Input: part model. Units: mm. Frame: model coordinates. Face numbers are marked on the shaded views. A direction names the side the tool comes from. Coordinates: 2 decimals unless noted, no trailing zeros. Write each loop counter-clockwise with the first axis right and the second up, starting at its lowest first coordinate (ties: lowest second). Pieces come first, ordered by that corner, then holes. Notation, with made-up numbers: M -24.5,-33.75 L -0.5,-33.75 A21 cw -0.5,4.25 Z; hole C 36,-36 d7. An arc over 180 degrees is marked long. Use one line per item in the form item = value.
from build123d import *

# Parameters (mm, degrees)
SKETCH1_R           = 3.1
SKETCH1_W           = 5.9
SKETCH1_H           = 5.9
BOSS_EXTRUDE1_DEPTH = 3.8
SKETCH2_W           = 5.9
SKETCH2_H           = 5.9
SKETCH2_R           = 1.7
BOSS_EXTRUDE2_DEPTH = 2
SKETCH3_R           = 3.1
BOSS_EXTRUDE3_DEPTH = 2
CHAMFER1_SIZE       = 0.5


with BuildPart() as part:
    # Sketch1 → Boss-Extrude1 (new body)
    with BuildSketch(Plane(origin=(0, 0, 0), x_dir=(1, 0, 0), z_dir=(0, 1, 0))):
        with BuildLine():
            Line((-5, 6.1), (5, 6.1))
            ThreePointArc((5, 6.1), (11.1, 0), (5, -6.1))
            Line((5, -6.1), (-5, -6.1))
            ThreePointArc((-5, -6.1), (-11.1, 0), (-5, 6.1))
        make_face()
        with Locations(Location((5, 0, 0), (0, 0, 90))):
            Circle(SKETCH1_R, mode=Mode.SUBTRACT)
        with Locations((-5, 0)):
            Rectangle(SKETCH1_W, SKETCH1_H, mode=Mode.SUBTRACT)
    extrude(amount=BOSS_EXTRUDE1_DEPTH)

    # Sketch2 → Boss-Extrude2 (add)
    with BuildSketch(Plane(origin=(0, 3.8, 0), x_dir=(1, 0, 0), z_dir=(0, 1, 0))):
        with Locations((-5, 0)):
            Rectangle(SKETCH2_W, SKETCH2_H)
        with Locations(Location((-5, 0, 0), (0, 0, 270))):
            Circle(SKETCH2_R, mode=Mode.SUBTRACT)
    extrude(amount=-BOSS_EXTRUDE2_DEPTH)

    # Sketch3 → Boss-Extrude3 (add)
    with BuildSketch(Plane.XZ):
        with Locations(Location((5, 0, 0), (0, 0, 270))):
            Circle(SKETCH3_R)
    extrude(amount=-BOSS_EXTRUDE3_DEPTH)

    # Chamfer1
    chamfer1_edges = [part.edges().sort_by_distance(p)[0] for p in [
        (5, 3.8, 3.1),
    ]]
    chamfer(chamfer1_edges, length=CHAMFER1_SIZE)


solid = part.part
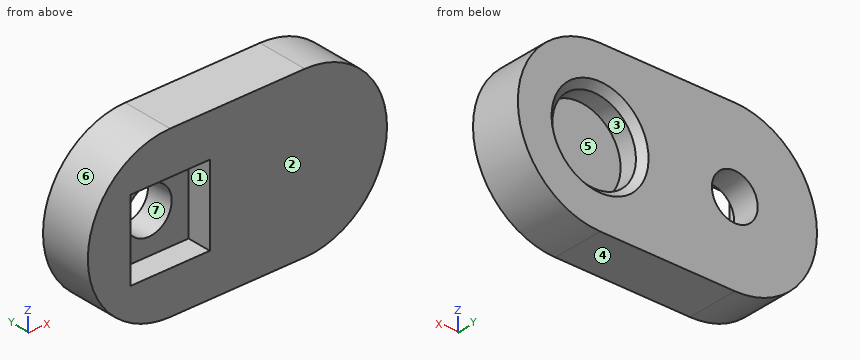
(1) Section query A-A on z = 0. Return the cut outline in (x, y), plus the area to 3 significant figures.
Computed:
outline = M -11.1,0 L -7.95,0 L -7.95,1.8 L -6.7,1.8 L -6.7,3.8 L -11.1,3.8 Z; M -3.3,1.8 L -2.05,1.8 L -2.05,0 L 11.1,0 L 11.1,3.8 L 8.6,3.8 L 8.1,3.3 L 8.1,2 L 1.9,2 L 1.9,3.3 L 1.4,3.8 L -3.3,3.8 Z
area = 55.5 mm^2
(2) Section query B-B on x = -4.25. Return the cut outline in (y, z).
Computed:
outline = M 0,-6.1 L 3.8,-6.1 L 3.8,-1.53 L 1.8,-1.53 L 1.8,-2.95 L 0,-2.95 Z; M 0,2.95 L 1.8,2.95 L 1.8,1.53 L 3.8,1.53 L 3.8,6.1 L 0,6.1 Z
(3) Section query C-C on y = 0.6. Return the cut outline in (x, z).
Computed:
outline = M -5,-6.1 L 5,-6.1 A6.1 ccw 5,6.1 L -5,6.1 A6.1 ccw Z; hole M -7.95,-2.95 L -2.05,-2.95 L -2.05,2.95 L -7.95,2.95 Z
(4) Set-up query: the marked faces 1, 2 and 3. Return all of +Z, -Z, +X, -X, +Y, -Y with unobstructed straight access to the full face (end or side cutting, diameter ignored); none if empty.
Computed:
face_1 = -Y
face_2 = +Z, -Z, +X, -X, -Y
face_3 = +Y
(5) Section query D-D on x = 9.25. Return the cut outline in (y, z), plus the area to 3 significant figures.
Computed:
outline = M 0,-4.38 L 3.8,-4.38 L 3.8,4.38 L 0,4.38 Z
area = 33.3 mm^2
(6) First-contact query: pin 1 Ø5 at (x, z) = (5, 0) entering from +Y; pin 2 Ø2 at (y, z) = (1, -1) entering from -X; pin 3 Ø4.5 at (x, z) = (-5, 0) entering from -Y; pin 4 Ø0.9 at (y, z) = (0.5, -1) entering from +X. Flat tips, straight axial feed; report the tip coordinate or a pass-through.
Computed:
pin_1 = 2
pin_2 = -11.1
pin_3 = 1.8
pin_4 = 11.08
(7) Line query: probe 1 along X at (y, z) = (2.4, 0); probe 2 along Z at (x, y) = (5, 2.9); probe 3 along X at (y, z) = (3.45, 0). Output: solid intervals per line, ascending.
Computed:
probe_1 = -11.1 to -6.7, -3.3 to 1.9, 8.1 to 11.1
probe_2 = -6.1 to -3.1, 3.1 to 6.1
probe_3 = -11.1 to -6.7, -3.3 to 1.75, 8.25 to 11.1
(8) Pull-direction query (Z, two-part tool) for the marked faces 4, 5, 6 and 7; classes: pulls with the +Z half, pulls with the -Z half, needs draft (parallel to the pull), parting line crosses it, or undercut.
Computed:
face_4 = pulls with the -Z half
face_5 = undercut
face_6 = parting line crosses it
face_7 = undercut
